Work out the finished part from the listing and answer in its coordinate system (mm). A direction names the side the tool comes from. Coordinates: 2 decimals unless noted, no trailing zeros. Loops run counter-clockwise (first coordinate to the right, second up) from the corner with the lowest first, then second, coordinate; pieces in that order, holes last. Notation, with made-up numbers: (87, -23.5) -> (134, -23.5) arc R26 ccw to (134, -8.5) -> close; hole circle Ø2 at (41.25, -35). An arc over 180 degrees is marked (long way). Answer as CSV lines item,"result".
```python
from build123d import *

# Parameters (mm, degrees)
F0_W      = 113
F0_H      = 64
F1_DEPTH  = 32
F2_W      = 32
F2_H      = 51
F3_DEPTH  = 25
F4_W      = 32
F4_H      = 51
F5_DEPTH  = 25
F7_DEPTH  = 32.001
F9_DEPTH  = 32.001
F10_SIZE  = 13
F11_SIZE  = 13
F12_R     = 5.5
F13_DEPTH = 13.001
F14_R     = 6.5
F15_DEPTH = 88.001


with BuildPart() as f1:
    # F0 (on Front) → F1 (new body)
    with BuildSketch(Plane.XZ):
        with Locations((-56.5, -32)):
            Rectangle(F0_W, F0_H)
    extrude(amount=F1_DEPTH)

    # F2 (on face) → F3 (cut)
    with BuildSketch(Plane.YZ):
        with Locations((-16, -25.5)):
            Rectangle(F2_W, F2_H)
    extrude(amount=-F3_DEPTH, mode=Mode.SUBTRACT)

    # F4 (on face) → F5 (cut)
    with BuildSketch(Plane(origin=(-113, 0, 0), x_dir=(0, -1, 0), z_dir=(-1, 0, 0))):
        with Locations((16, -25.5)):
            Rectangle(F4_W, F4_H)
    extrude(amount=-F5_DEPTH, mode=Mode.SUBTRACT)

    # F6 (on face) → F7 (cut, through all)
    with BuildSketch(Plane.XZ.offset(32)):
        Polygon((-39, -47), (-56.5, -47), (-74, -47), (-74, -64), (-56.5, -64), (-39, -64), align=None)
    extrude(amount=-F7_DEPTH, mode=Mode.SUBTRACT)

    # F8 (on face) → F9 (cut, through all)
    with BuildSketch(Plane.XZ.offset(32)):
        Polygon((-69, -34), (-56.5, -34), (-44, -34), (-44, 0), (-56.5, 0), (-69, 0), align=None)
    extrude(amount=-F9_DEPTH, mode=Mode.SUBTRACT)

    # F10
    f10_edges = [f1.edges().sort_by_distance(p)[0] for p in [
        (-113, -32, -57.5),
    ]]
    chamfer(f10_edges, length=F10_SIZE)

    # F11
    f11_edges = [f1.edges().sort_by_distance(p)[0] for p in [
        (0, -32, -57.5),
    ]]
    chamfer(f11_edges, length=F11_SIZE)

    # F12 (on face) → F13 (cut, through all)
    with BuildSketch(Plane.XY.offset(-51)):
        with Locations((-100.480012, -12.999985)):
            Circle(F12_R)
        with Locations((-13, -13)):
            Circle(F12_R)
    extrude(amount=-F13_DEPTH, mode=Mode.SUBTRACT)

    # F14 (on face) → F15 (cut, through all)
    with BuildSketch(Plane.YZ.offset(-25)):
        with Locations((-15.079716, -18)):
            Circle(F14_R)
    extrude(amount=-F15_DEPTH, mode=Mode.SUBTRACT)


solid = f1.part
```
(1) A cutting plane is placed at D-D, the plane x = -72. Write down the section's boundary in (y, z), and give its area (3 significant figures).
Computed values:
outline,"(-32, -47) -> (0, -47) -> (0, 0) -> (-32, 0) -> close; hole circle Ø13 at (-15.08, -18)"
area,"1,370 mm2"
(2) A cutting plane is placed at C-C, the plane z = -28. Write down the section's boundary in (x, y), and give its area (3 significant figures).
Computed values:
outline,"(-88, -32) -> (-69, -32) -> (-69, 0) -> (-88, 0) -> close; (-44, -32) -> (-25, -32) -> (-25, 0) -> (-44, 0) -> close"
area,"1,220 mm2"
(3) A cutting plane is placed at B-B, the plane x = -102. Write down the section's boundary in (y, z), and give its area (3 significant figures).
Computed values:
outline,"(-30, -64) -> (-18.29, -64) -> (-18.29, -51) -> (-30, -51) -> close; (-7.71, -64) -> (0, -64) -> (0, -51) -> (-7.71, -51) -> close"
area,"253 mm2"
(4) Flat-ended cylindrical pins translate along their axes: pin 1 Ø7.5 at (x, y) = (-61, -24) entering from +Z; pin 2 Ø1 at (y, z) = (-8.5, -25) entering from +X; pin 3 Ø12.5 at (x, y) = (-105.5, -11.5) entering from +Z; pin 4 Ø6.5 at (x, y) = (-13, -13) entering from -Z. Find the tip coordinate at first contact, or state that the pin passes through.
Computed values:
pin 1,"z = -34"
pin 2,"x = -25"
pin 3,"z = -51"
pin 4,"through"
(5) Which of the six approach directions +Z, -Z, +X, -X, +Y, -Y give full straight-line access (tool end or side, diameter ignored) to faces 4 (the face through (-69, -20, -13)), 5 (the face through (-101, -19, -51)), 6 (the face through (-34.367, -19.87, -13.607)), 7 (the face through (-25, -16, -25))?
Computed values:
face 4,"+Z, +Y, -Y"
face 5,"+Z, -X, +Y, -Y"
face 6,"+X, -X"
face 7,"+Z, +X, +Y, -Y"
(6) For a pull along Y with two mould halves and no side action, classify faces 1 (the face through (-20, -16, -64)), 2 (the face through (-105.975, -12.758, -57.409)), 3 (the face through (-57, -32, -39)) as pulls with the +Y half, pulls with the -Y half, needs draft (parallel to the pull), parting line crosses it, or undercut.
Computed values:
face 1,"needs draft"
face 2,"undercut"
face 3,"pulls with the -Y half"
(7) Consider line 1 along X through (y, z) = (-16.5, -28.5); line 2 along X through (y, z) = (-9.5, -60.5); line 3 along X through (y, z) = (-2.5, -55). Determine where each line is inside the solid, lowest interval first.
Computed values:
line 1,"-88 to -69, -44 to -25"
line 2,"-113 to -104.72, -96.24 to -74, -39 to -17.24, -8.76 to 0"
line 3,"-113 to -74, -39 to 0"
(8) A cutting plane is placed at A-A, the plane z = -18. Write down the section's boundary in (x, y), and give its area (3 significant figures).
Computed values:
outline,"(-88, -32) -> (-69, -32) -> (-69, -21.58) -> (-88, -21.58) -> close; (-88, -8.58) -> (-69, -8.58) -> (-69, 0) -> (-88, 0) -> close; (-44, -32) -> (-25, -32) -> (-25, -21.58) -> (-44, -21.58) -> close; (-44, -8.58) -> (-25, -8.58) -> (-25, 0) -> (-44, 0) -> close"
area,"722 mm2"
